Could you check a few things on this model? Use its own coordinates, in mm. A direction names the side the tool comes from. Round coordinates to 2 decimals unless told otherwise and drop trailing zeros. Order: outer loops, then holes, each group sorted by start corner. A loop starts at its lowest first (then second) coordinate and runs counter-clockwise, first axis right, second up. Notation, with made-up numbers: (58, 47) - (91, 47) arc R10 cw to (91, 59) - close; hole circle Ø4 at (43, 38.25). An arc over 180 degrees is marked (long way). Use one line per item in the form item = value.
from build123d import *

# Parameters (mm, degrees)
SKETCH_4_R      = 8.137661996
SKETCH_4_W      = 31.9414987
SKETCH_4_H      = 36.578678147
EXTRUDE_1_DEPTH = 10


with BuildPart() as part:
    # 草图4 → 凸台-拉伸1 (new body)
    with BuildSketch(Plane.XY):
        Polygon((-115.679167542, 163.709819989), (-112.783171997, 167.977826386), (-112.783171997, 172.521825104), (-135.13516787, 172.401821332), (-135.13516787, 163.073818402), (-145.12317358, 163.073823243), (-145.12317358, 151.265824585), (-135.13516787, 151.265819745), (-135.13516787, 127.321818547), (-145.12317358, 127.321823388), (-145.12317358, 115.485822707), (-135.13517271, 115.485822707), (-135.13517271, 96.149821549), (-145.123168739, 96.149816708), (-145.123168739, 84.229816632), (-135.13516787, 84.229816632), (-135.13516787, 60.175815779), (-145.121572289, 60.175815779), (-145.121564659, 48.342350203), (-135.13516024, 48.342350203), (-135.135152611, 24.396549422), (-145.121564659, 24.396549422), (-145.12155703, 12.587940413), (-135.135152611, 12.587940413), (-135.135152611, 3.261310774), (-131.182853493, 3.139713484), (-131.182853493, -12.691325945), (-120.512386116, -12.691325945), (-120.512386116, -53.276546281), (-135.177665504, -53.276546281), (-135.177665504, -56.177557678), (-145.201591286, -56.177547258), (-145.201591286, -60.195171159), (-135.177670343, -60.195181579), (-135.177670343, -63.017477722), (-126.064049585, -65.69681427), (-111.259845528, -73.199390215), (-110.188045296, -74.539134782), (-110.18804911, -87.630618852), (-135.177657875, -87.630618852), (-135.177657875, -91.900821489), (-145.201591286, -91.900821489), (-145.201591286, -103.616760057), (-135.177657875, -103.616760057), (-135.177657875, -109.910648149), (-112.782481941, -110.032245439), (-112.782471521, -105.487982482), (-115.679146631, -101.218363494), (-97.719758046, -101.218377487), (-100.181937965, -105.487979692), (-100.181937965, -110.032241624), (-78.482952936, -109.910639495), (-78.482950005, -103.616755218), (-68.496559961, -103.616759033), (-68.496559961, -91.90081665), (-78.482960566, -91.90081665), (-78.482959541, -27.976309509), (-68.496556147, -27.976309509), (-68.496556147, -16.124869079), (-78.482955727, -16.124869079), (-78.48294619, 13.220635682), (-68.49654661, 13.220635682), (-68.496550425, 24.47091034), (-78.482954844, 24.47091034), (-78.482957634, 48.412209778), (-68.496554239, 48.412209778), (-68.496558054, 60.263650208), (-78.482957634, 60.263650208), (-78.495166571, 84.237820893), (-68.499169214, 84.237820893), (-68.499169214, 96.109822541), (-78.495171412, 96.109822541), (-78.495171412, 105.761817174), (-68.499164374, 105.761817174), (-68.499164374, 115.473818021), (-78.495171412, 115.473822861), (-78.495171412, 151.265819745), (-68.499164374, 151.265819745), (-68.499169214, 163.073823243), (-78.495166573, 163.073818402), (-78.495166573, 172.401821332), (-100.183171615, 172.521825104), (-100.183171615, 167.977826386), (-97.72316626, 163.709819989), align=None)
        with Locations((-99.461505196, 103.795957581)):
            Circle(SKETCH_4_R, mode=Mode.SUBTRACT)
        Polygon((-110.230805262, -12.691321106), (-90.593654427, -12.691325945), (-90.593668373, -78.776897231), (-110.230815681, -62.066013139), align=None, mode=Mode.SUBTRACT)
        with Locations((-106.564418137, 57.028483651)):
            Rectangle(SKETCH_4_W, SKETCH_4_H, mode=Mode.SUBTRACT)
        Polygon((-119.863172396, 153.513820843), (-94.943171363, 153.621818753), (-94.943166525, 125.645818429), (-119.863172396, 118.361822902), align=None, mode=Mode.SUBTRACT)
    extrude(amount=EXTRUDE_1_DEPTH)


solid = part.part
Item 1: If we mould it in two halves opening along X, with no side actions, what happens to faces 5 (the face through (-107, 75.318, 5)), 6 (the face through (-119.863, 136, 5)), 7 (the face through (-78.483, -2, 5)), 8 (the face through (-73, 96.11, 5))? For each: released by +X, released by -X, zero draft, split by the parting line, or undercut.
Found:
face_5 = undercut
face_6 = undercut
face_7 = released by +X
face_8 = zero draft
Item 2: Imagine slicing it at D-D on z = 7.5. State how many separate pieces and enclosed holes the cut face has, plus the area to 3 significant figures.
Found:
separate_pieces = 1
enclosed_holes = 4
area = 12,900 mm2
Item 3: Imagine slicing it at C-C on x = -104. Please give me the cut outline in (y, z).
Found:
outline = (-101.22, 0) - (-67.37, 0) - (-67.37, 10) - (-101.22, 10) - close; (-12.69, 0) - (38.74, 0) - (38.74, 10) - (-12.69, 10) - close; (75.32, 0) - (97.04, 0) - (97.04, 10) - (75.32, 10) - close; (110.55, 0) - (123, 0) - (123, 10) - (110.55, 10) - close; (153.58, 0) - (163.71, 0) - (163.71, 10) - (153.58, 10) - close
Item 4: I need wall thicknesses on L1, parallel to X at y = 61.5, z = 7.5; L2, parallel to Y at x = -95.5, z = 3.5; L3, parallel to Y at x = -127.5, z = 0.5. Which ranges of each line are inside material? Lowest first, please.
Found:
L1 = -135.14 to -122.54, -90.59 to -78.48
L2 = -110.01 to -74.6, -12.69 to 38.74, 75.32 to 96.69, 110.9 to 125.48, 153.62 to 172.5
L3 = -109.95 to -87.63, -65.27 to -53.28, -12.69 to 172.44
Item 5: Will these pins go through, and if not, where does the flat tip stop? P1, Ø6, axis at y = -71.5, z = 2.5, coming from the +X side; P2, Ø3, axis at x = -102.5, z = 6, coming from the -Y side; P3, Ø5, axis at y = -106.5, z = 6.5, coming from the -X side.
Found:
P1 = -78.48
P2 = -101.22
P3 = -135.18
Item 6: Imagine slicing it at B-B on x = -73.5. Please give me the cut outline in (y, z).
Found:
outline = (-103.62, 0) - (-91.9, 0) - (-91.9, 10) - (-103.62, 10) - close; (-27.98, 0) - (-16.12, 0) - (-16.12, 10) - (-27.98, 10) - close; (13.22, 0) - (24.47, 0) - (24.47, 10) - (13.22, 10) - close; (48.41, 0) - (60.26, 0) - (60.26, 10) - (48.41, 10) - close; (84.24, 0) - (96.11, 0) - (96.11, 10) - (84.24, 10) - close; (105.76, 0) - (115.47, 0) - (115.47, 10) - (105.76, 10) - close; (151.27, 0) - (163.07, 0) - (163.07, 10) - (151.27, 10) - close
Item 7: For faces 1 (the face through (-73, 163.074, 5)), 2 (the face through (-135.135, 72, 5)), 3 (the face through (-140, 163.074, 5)), 4 (the face through (-74, 151.266, 5)), which set-ups out of +Z, -Z, +X, -X, +Y, -Y let a thin tool reach every point of the face, with its end or its side?
Found:
face_1 = +Z, -Z, +X, +Y
face_2 = +Z, -Z, -X
face_3 = +Z, -Z, -X, +Y
face_4 = +Z, -Z, +X
Item 8: Imagine slicing it at A-A on y = -46. Please give me the cut outline in (x, z), plus the area to 3 significant figures.
Found:
outline = (-120.51, 0) - (-110.23, 0) - (-110.23, 10) - (-120.51, 10) - close; (-90.59, 0) - (-78.48, 0) - (-78.48, 10) - (-90.59, 10) - close
area = 224 mm2
